Read the model definition and answer for the solid it produces. Units are mm, in the model's axes. A direction names the side the tool comes from. Coordinates: 2 decimals unless noted, no trailing zeros. Order: outer loops, then holes, each group sorted by start corner. A loop starts at its lowest first (then second) coordinate and runs counter-clockwise, first axis right, second up. Notation, with made-up numbers: M 4,28 L 39,28 A15 ccw 39,50 Z; hole C 89.25,-4 d7. An arc over 180 degrees is marked long. Use a Markdown table: item, result. Add a question column.
1) Find section C-C on y = 27. Write down the section's boundary in (x, z), plus the area to 3 significant figures.
2) For faces 5 (the face through (24, 4, 0)), 6 (the face through (-12.5, 26, 0)), 7 (the face through (12.5, 26, 0)), determine the directions among +Z, -Z, +X, -X, +Y, -Y from which every point of the face is accessible in a straight line to the end or side of a thin tool.
3) Each of these flat-tipped pins is pushed along its axis until it touches: pin 1 Ø8 at (y, z) = (13.5, -5.5) entering from +X; pin 2 Ø9 at (x, z) = (18.5, 0) entering from +Y; pin 3 Ø6 at (y, z) = (20, 3) entering from -X. Where does it stop, or does it pass through?
4) Find the intervals of material crossed by probe 1 along X at (y, z) = (2.75, 0); probe 2 along Z at (x, y) = (-19, 3.5); probe 3 along Y at (x, z) = (0, -0.5), in increasing order. Write a range as [from, to].
5) Find section B-B on z = 0. Write down the section's boundary in (x, y).
6) Find section D-D on z = -6.75. Write down the section's boundary in (x, y).
7) Find section A-A on x = 0. Write down the section's boundary in (y, z), plus the area to 3 significant figures.
8) The mould has two halves that part along Z. Classify faces 1 (the face through (-21.727, 4.056, 0.358)), 2 (the face through (0, 44, 0)), 3 (the face through (21.727, 4.056, -0.358)), 4 (the face through (0, 17, 8)): released by +Z, released by -Z, zero draft, split by the parting line, or undercut.
from build123d import *

# Parameters (mm, degrees)
SKETCH_1_R          = 8
EXTRUDE_1_DEPTH     = 8
SKETCH_2_R          = 2.75
CUT_EXTRUDE_1_DEPTH = 45


with BuildPart() as part:
    # 草图1 → 凸台-拉伸1 (new, symmetric)
    with BuildSketch(Plane.XY):
        Polygon((-24, 0), (24, 0), (24, 8), (12.5, 8), (12.5, 44), (-12.5, 44), (-12.5, 8), (-24, 8), align=None)
        with Locations((0, 27)):
            Circle(SKETCH_1_R, mode=Mode.SUBTRACT)
    extrude(amount=EXTRUDE_1_DEPTH, both=True)

    # 草图2 → 切除-拉伸1 (cut, through all)
    with BuildSketch(Plane(origin=(0, 8, 0), x_dir=(1, 0, 0), z_dir=(0, 1, 0))):
        with Locations(Location((19, 0, 0), (0, 0, 270))):
            Circle(SKETCH_2_R)
        with Locations(Location((-19, 0, 0), (0, 0, 90))):
            Circle(SKETCH_2_R)
    extrude(amount=-CUT_EXTRUDE_1_DEPTH, mode=Mode.SUBTRACT)


solid = part.part
Check result:
| question | item | result |
|---|---|---|
| 1 | outline | M -12.5,-8 L -8,-8 L -8,8 L -12.5,8 Z; M 8,-8 L 12.5,-8 L 12.5,8 L 8,8 Z |
| 1 | area | 144 mm2 |
| 2 | face 5 | +Z, -Z, +X, +Y, -Y |
| 2 | face 6 | +Z, -Z, -X, +Y |
| 2 | face 7 | +Z, -Z, +X, +Y |
| 3 | pin 1 | stops at x = 12.5 |
| 3 | pin 2 | stops at y = 8 |
| 3 | pin 3 | stops at x = -12.5 |
| 4 | probe 1 | x = [-24, -21.75], [-16.25, 16.25], [21.75, 24] |
| 4 | probe 2 | z = [-8, -2.75], [2.75, 8] |
| 4 | probe 3 | y = [0, 19], [35, 44] |
| 5 | outline | M -24,0 L -21.75,0 L -21.75,8 L -24,8 Z; M -16.25,0 L 16.25,0 L 16.25,8 L 12.5,8 L 12.5,44 L -12.5,44 L -12.5,8 L -16.25,8 Z; M 21.75,0 L 24,0 L 24,8 L 21.75,8 Z; hole C 0,27 d16 |
| 6 | outline | M -24,0 L 24,0 L 24,8 L 12.5,8 L 12.5,44 L -12.5,44 L -12.5,8 L -24,8 Z; hole C 0,27 d16 |
| 7 | outline | M 0,-8 L 19,-8 L 19,8 L 0,8 Z; M 35,-8 L 44,-8 L 44,8 L 35,8 Z |
| 7 | area | 448 mm2 |
| 8 | face 1 | undercut |
| 8 | face 2 | zero draft |
| 8 | face 3 | undercut |
| 8 | face 4 | released by +Z |
